Part print with two shaded views. Sizes in mm from the minimum x, y, z corner. Give positions to 0.01 mm unless a question says otherwise; leave off trailing zeros. Write each loop counter-clockwise with the first axis right and the second up, starting at its lowest first coordinate (ties: lowest second). Pieces come first, ordered by that corner, then holes. Notation, with made-up numbers: M -4.5,15.5 L 43.5,15.5 A17 cw 43.5,19.5 Z; hole C 5.25,37 d3. An arc over 180 degrees is marked long. Return JSON: item names as keys, results as strings. Group by question number.
Q1. Band-saw the part on A-A, the plane x = 49. Give the cut face in (y, z).
Q2. Band-saw the part on D-D, the plane z = 18.25. Give the cut face in (x, y).
Q3. Flat gauge pins, fed straight in: pin 1 Ø1.5 at (x, y) = (83, 1) entering from -Z; pin 2 Ø2.5 at (x, z) = (25.5, 66.5) entering from +Y. Where does each tip first touch, or does it go through?
Q4. Wall check: probe 1 along Z at (x, y) = (45.5, 0.8); probe 2 along Z at (x, y) = (104.5, 1.8); probe 3 along X at (y, z) = (1, 66.5). Give the ranges that are in metal, low to high.
Q5. Band-saw the part on B-B, the plane z = 4.5. Give the cut face in (x, y).
Q6. Band-saw the part on C-C, the plane x = 104.5. Give the cut face in (y, z), then the cut area to 3 significant figures.
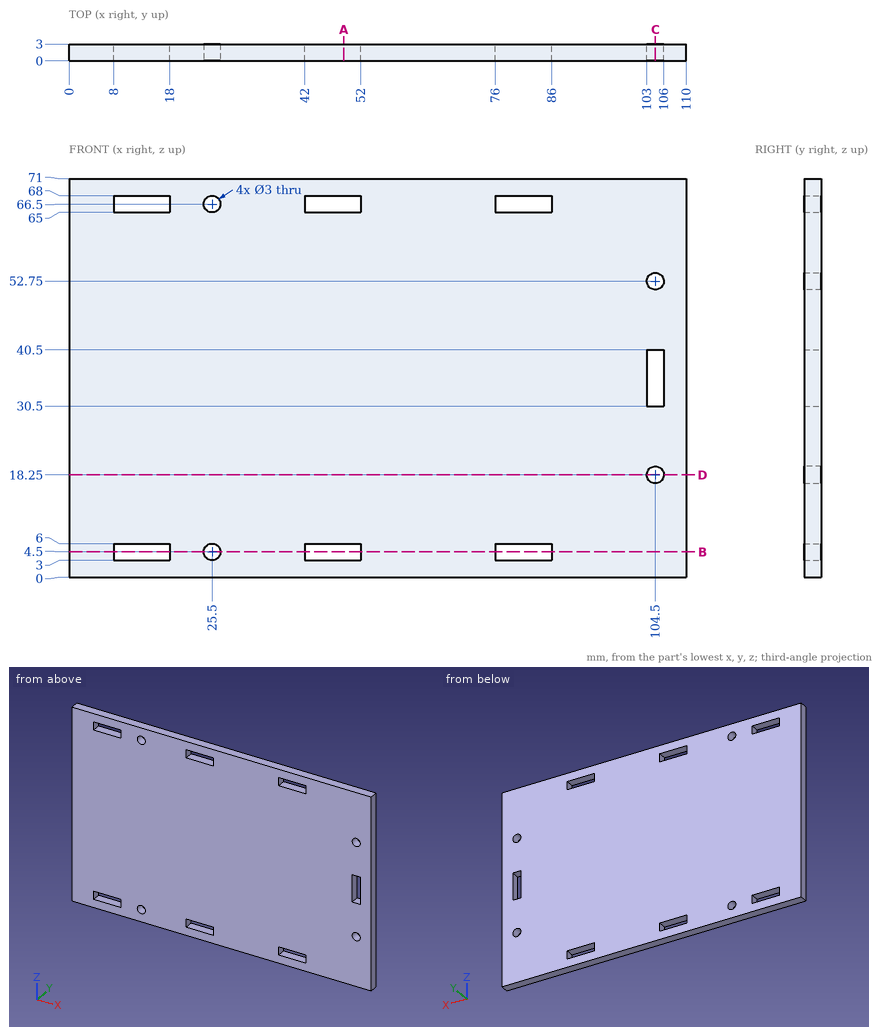
From the geometry:
{
 "1": {"outline": "M 0,0 L 3,0 L 3,3 L 0,3 Z; M 0,6 L 3,6 L 3,65 L 0,65 Z; M 0,68 L 3,68 L 3,71 L 0,71 Z"},
 "2": {"outline": "M 0,0 L 103,0 L 103,3 L 0,3 Z; M 106,0 L 110,0 L 110,3 L 106,3 Z"},
 "3": {"pin 1": "stops at z = 0", "pin 2": "passes through"},
 "4": {"probe 1": "z = 0 to 3, 6 to 65, 68 to 71", "probe 2": "z = 0 to 16.75, 19.75 to 30.5, 40.5 to 51.25, 54.25 to 71", "probe 3": "x = 0 to 8, 18 to 24, 27 to 42, 52 to 76, 86 to 110"},
 "5": {"outline": "M 0,0 L 8,0 L 8,3 L 0,3 Z; M 18,0 L 24,0 L 24,3 L 18,3 Z; M 27,0 L 42,0 L 42,3 L 27,3 Z; M 52,0 L 76,0 L 76,3 L 52,3 Z; M 86,0 L 110,0 L 110,3 L 86,3 Z"},
 "6": {"outline": "M 0,0 L 3,0 L 3,16.75 L 0,16.75 Z; M 0,19.75 L 3,19.75 L 3,30.5 L 0,30.5 Z; M 0,40.5 L 3,40.5 L 3,51.25 L 0,51.25 Z; M 0,54.25 L 3,54.25 L 3,71 L 0,71 Z", "area": "165 mm^2"}
}
